Check sheet for the modelled part. Datum: model origin and axes. Units: mm. Face numbers are marked on the shaded views. A direction names the side the tool comes from. Give positions to 0.01 mm unless a question says otherwise; leave off trailing zeros. Loops run counter-clockwise (first coordinate to the right, second up) from the corner with the lowest first, then second, coordinate; pieces in that order, holes last. Notation, with made-up numbers: M 77,-23.75 L 81,-23.75 A23 cw 81,3.25 Z; hole C 34.25,46 d2. An arc over 180 degrees is marked long. Write each question's results on one line, items separated by ' | '. Start each with the question number.
1. Sectioned sample at B-B on x = 7.5. Record the cut outline in (y, z).
2. Material ranges on line 1 along Y through (x, z) = (-16.75, 7.25) (3 decimals); line 2 along Y through (x, z) = (-16, 12); line 3 along X through (y, z) = (9.75, 5.5), recorded low to high.
3. Sectioned sample at A-A on x = -16.75. Record the cut outline in (y, z) (3 decimals), and give its area (3 significant figures).
4. Sectioned sample at D-D on z = 13. Give the number of separate pieces and of enclosed holes in the cut face, and give its area (3 significant figures).
5. Go/stop test with flat-tipped pins: pin 1 (3 mm diameter, centred on x = 7.5, z = -5.5, fed in from -Y); pin 2 (1.6 mm diameter, centred on x = 16.75, y = -9.47, fed in from +Z); pin 3 (3 mm diameter, centred on x = -7, y = 3, fed in from +Z); pin 4 (8 mm diameter, centred on x = -26.5, z = 2.5, fed in from -Y). Record where each tip stops, or that it passes through.
6. Sectioned sample at C-C on z = 21.5. Record the cut outline in (x, y), and give its area (3 significant figures).
7. Tool access check on the marked faces 1, 2 and 3. Record the directions out of +Z, -Z, +X, -X, +Y, -Y that give a thin tool (end or side, any length) a straight path to the whole face; none if there is none.
```python
from build123d import *

# Parameters (mm, degrees)
SKETCH1_W                = 37
SKETCH1_H                = 22.44
BOSS_EXTRUDE1_DEPTH      = 18.6
FILLET1_R                = 2
SKETCH2_W                = 17
SKETCH2_H                = 20.38
BOSS_EXTRUDE2_DEPTH      = 14
BOSS_EXTRUDE3_DEPTH      = 9.3
BOSS_EXTRUDE3_DEPTH_BACK = 26.7
CUT_EXTRUDE1_DEPTH       = 14
SKETCH5_R                = 0.975
CUT_EXTRUDE2_DEPTH       = 45.278080455


with BuildPart() as part:
    # Sketch1 → Boss-Extrude1 (new body)
    with BuildSketch(Plane.XY):
        Rectangle(SKETCH1_W, SKETCH1_H)
    extrude(amount=BOSS_EXTRUDE1_DEPTH)

    # Fillet1
    fillet1_edges = [part.edges().sort_by_distance(p)[0] for p in [
        (18.5, 11.22, 9.3),
        (18.5, -11.22, 9.3),
    ]]
    fillet(fillet1_edges, radius=FILLET1_R)

    # Sketch2 → Boss-Extrude2 (add)
    with BuildSketch(Plane.ZY.offset(18.5)):
        with Locations((9.3, 0)):
            Rectangle(SKETCH2_W, SKETCH2_H)
    extrude(amount=BOSS_EXTRUDE2_DEPTH)

    # Sketch3 → Boss-Extrude3 (add, two sides: drawn at the far end of the back side and taken through both)
    with BuildSketch(Plane.XY.offset(18.6).offset(-BOSS_EXTRUDE3_DEPTH_BACK)):
        with BuildLine():
            Line((5.533403956, 1.85), (9.466596044, 1.85))
            ThreePointArc((9.466596044, 1.85), (10.2, 0), (9.466596044, -1.85))
            Line((9.466596044, -1.85), (5.533403956, -1.85))
            ThreePointArc((5.533403956, -1.85), (4.8, 0), (5.533403956, 1.85))
        make_face()
    extrude(amount=BOSS_EXTRUDE3_DEPTH + BOSS_EXTRUDE3_DEPTH_BACK)

    # Sketch4 → Cut-Extrude1 (cut)
    with BuildSketch(Plane.ZY.offset(32.5)):
        with BuildLine():
            Line((0.8, 10.19), (0.8, 0.135437192))
            add(Edge.make_bspline(
                [(9.236397672, 10.19), (0.95810585, 10.058115826), (0.8, 0.135437192)],
                knots=[0.026580808, 0.026580808, 0.026580808, 1.570796327, 1.570796327, 1.570796327], degree=2, weights=[1, 0.71644179, 1]))
            Line((9.236397672, 10.19), (0.8, 10.19))
        make_face()
        with BuildLine():
            Line((17.8, 10.19), (9.462365292, 10.19))
            add(Edge.make_bspline(
                [(17.8, 0.25381428), (17.64372138, 10.059640013), (9.462365292, 10.19)],
                knots=[4.750587933, 4.750587933, 4.750587933, 6.283185307, 6.283185307, 6.283185307], degree=2, weights=[1, 0.72048236, 1]))
            Line((17.8, 0.25381428), (17.8, 10.19))
        make_face()
        with BuildLine():
            add(Edge.make_bspline(
                [(9.363602328, -10.19), (17.64189415, -10.058115826), (17.8, -0.135437192)],
                knots=[3.168173462, 3.168173462, 3.168173462, 4.71238898, 4.71238898, 4.71238898], degree=2, weights=[1, 0.71644179, 1]))
            Line((9.363602328, -10.19), (17.8, -10.19))
            Line((17.8, -10.19), (17.8, -0.135437192))
        make_face()
        with BuildLine():
            add(Edge.make_bspline(
                [(0.8, -0.25381428), (0.95627862, -10.059640013), (9.137634708, -10.19)],
                knots=[1.608995279, 1.608995279, 1.608995279, 3.141592654, 3.141592654, 3.141592654], degree=2, weights=[1, 0.72048236, 1]))
            Line((0.8, -0.25381428), (0.8, -10.19))
            Line((0.8, -10.19), (9.137634708, -10.19))
        make_face()
    extrude(amount=-CUT_EXTRUDE1_DEPTH, mode=Mode.SUBTRACT)

    # Sketch5 → Cut-Extrude2 (cut, through all)
    with BuildSketch(Plane(origin=(0, 0, 0), x_dir=(-1, 0, 0), z_dir=(0, 0, -1))):
        with Locations((-16.75, 9.47)):
            Circle(SKETCH5_R)
        with Locations((-16.75, -9.47)):
            Circle(SKETCH5_R)
        with Locations((16.75, -9.47)):
            Circle(SKETCH5_R)
        with Locations((16.75, 9.47)):
            Circle(SKETCH5_R)
    extrude(amount=-CUT_EXTRUDE2_DEPTH, mode=Mode.SUBTRACT)


solid = part.part
```
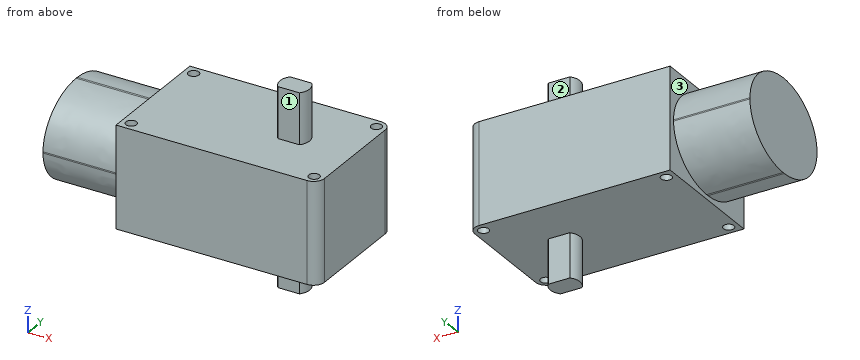
Output values:
1) outline: M -11.22,0 L -1.85,0 L -1.85,-8.1 L 1.85,-8.1 L 1.85,0 L 11.22,0 L 11.22,18.6 L 1.85,18.6 L 1.85,27.9 L -1.85,27.9 L -1.85,18.6 L -11.22,18.6 Z
2) line 1: -11.22 to -10.445, -8.495 to 8.495, 10.445 to 11.22 | line 2: -11.22 to -10.09, -8.85 to 8.85, 10.09 to 11.22 | line 3: -18.5 to -17.68, -15.82 to 15.82, 17.68 to 18.43
3) outline: M -11.22,0 L -10.445,0 L -10.445,18.6 L -11.22,18.6 Z; M -8.495,0 L 8.495,0 L 8.495,18.6 L -8.495,18.6 Z; M 10.445,0 L 11.22,0 L 11.22,18.6 L 10.445,18.6 Z | area: 345 mm2
4) separate pieces: 1 | enclosed holes: 4 | area: 1,070 mm2
5) pin 1: y = -1.85 | pin 2: through | pin 3: z = 18.6 | pin 4: y = -9.64
6) outline: M 5.53,-1.85 L 9.47,-1.85 A2.7 ccw 9.47,1.85 L 5.53,1.85 A2.7 ccw Z | area: 18.3 mm2
7) face 1: +Z, +X, -X, -Y | face 2: +Z, +X, -X, +Y | face 3: -X
